from build123d import *

# Parameters (mm, degrees)
F0_R     = 1.2
F0_R_2   = 2.05
F1_DEPTH = 5.6
F2_R     = 1.6
F2_R_2   = 2.45
F3_DEPTH = 25


with BuildPart() as f1:
    # F0 (on Top) → F1 (new body)
    with BuildSketch(Plane.XY):
        with BuildLine():
            Line((31.5, 25.5), (39.5, 25.5))
            Line((39.5, 25.5), (39.5, 44.5))
            Line((39.5, 44.5), (22.808842361, 61.3844171166))
            Line((22.808842361, 61.3844171166), (0, 61.3844171166))
            Line((0, 61.3844171166), (-22.808842361, 61.3844171166))
            Line((-22.808842361, 61.3844171166), (-39.5, 44.5))
            Line((-39.5, 44.5), (-39.5, 25.5))
            Line((-39.5, 25.5), (-31.5, 25.5))
            Line((-31.5, 25.5), (-31.5, 18.901754251))
            ThreePointArc((-31.5, 18.901754251), (0, 41), (31.5, 18.901754251))
            Line((31.5, 18.901754251), (31.5, 25.5))
        make_face()
        with Locations((-35, 43)):
            Circle(F0_R, mode=Mode.SUBTRACT)
        with Locations((0, 54.8844171166)):
            Circle(F0_R_2, mode=Mode.SUBTRACT)
        with Locations((35, 43)):
            Circle(F0_R, mode=Mode.SUBTRACT)
        with BuildLine():
            Line((22.808842361, -61.3844171166), (39.5, -44.5))
            Line((39.5, -44.5), (39.5, -9.5))
            Line((39.5, -9.5), (31.5, -9.5))
            Line((31.5, -9.5), (31.5, -3.901754251))
            ThreePointArc((31.5, -3.901754251), (0, -26), (-31.5, -3.901754251))
            Line((-31.5, -3.901754251), (-31.5, -9.5))
            Line((-31.5, -9.5), (-39.5, -9.5))
            Line((-39.5, -9.5), (-39.5, -44.5))
            Line((-39.5, -44.5), (-22.808842361, -61.3844171166))
            Line((-22.808842361, -61.3844171166), (0, -61.3844171166))
            Line((0, -61.3844171166), (22.808842361, -61.3844171166))
        make_face()
        with Locations((-35, -43)):
            Circle(F0_R, mode=Mode.SUBTRACT)
        with Locations((0, -54.8844171166)):
            Circle(F0_R_2, mode=Mode.SUBTRACT)
        with Locations((35, -43)):
            Circle(F0_R, mode=Mode.SUBTRACT)
        with BuildLine():
            Line((-31.5, -9.5), (-31.5, -3.901754251))
            ThreePointArc((-31.5, -3.901754251), (-33.5, 7.5), (-31.5, 18.901754251))
            Line((-31.5, 18.901754251), (-31.5, 25.5))
            Line((-31.5, 25.5), (-39.5, 25.5))
            Line((-39.5, 25.5), (-39.5, -9.5))
            Line((-39.5, -9.5), (-31.5, -9.5))
        make_face()
        with BuildLine():
            Line((31.5, -9.5), (39.5, -9.5))
            Line((39.5, -9.5), (39.5, 25.5))
            Line((39.5, 25.5), (31.5, 25.5))
            Line((31.5, 25.5), (31.5, 18.901754251))
            ThreePointArc((31.5, 18.901754251), (32.9962119038, 13.2879184514), (33.5, 7.5))
            ThreePointArc((33.5, 7.5), (32.9962119038, 1.7120815486), (31.5, -3.901754251))
            Line((31.5, -3.901754251), (31.5, -9.5))
        make_face()
    extrude(amount=F1_DEPTH)

    # F2 (on face) → F3 (cut)
    with BuildSketch(Plane.XY.offset(5.6)):
        with Locations((-31, 38.5)):
            Circle(F2_R)
        with Locations((31, 38.5)):
            Circle(F2_R)
        with Locations((-31, -23.5)):
            Circle(F2_R)
        with Locations((31, -23.5)):
            Circle(F2_R)
        with Locations((0, 54.8844171166)):
            Circle(F2_R_2)
        with Locations((0, -54.8844171166)):
            Circle(F2_R_2)
        with BuildLine():
            ThreePointArc((10.5, 56.3844171166), (10.0606601718, 57.4450772884), (9, 57.8844171166))
            Line((9, 57.8844171166), (9, 54.8844171166))
            ThreePointArc((9, 54.8844171166), (10.0606601718, 55.3237569449), (10.5, 56.3844171166))
        make_face()
        with BuildLine():
            Line((17, 57.8844171166), (9, 57.8844171166))
            ThreePointArc((9, 57.8844171166), (10.0606601718, 57.4450772884), (10.5, 56.3844171166))
            ThreePointArc((10.5, 56.3844171166), (10.0606601718, 55.3237569449), (9, 54.8844171166))
            Line((9, 54.8844171166), (17, 54.8844171166))
            ThreePointArc((17, 54.8844171166), (15.5, 56.3844171166), (17, 57.8844171166))
        make_face()
        with BuildLine():
            Line((9, 54.8844171166), (9, 57.8844171166))
            ThreePointArc((9, 57.8844171166), (7.5, 56.3844171166), (9, 54.8844171166))
        make_face()
        with BuildLine():
            ThreePointArc((18.5, 56.3844171166), (18.0606601718, 57.4450772884), (17, 57.8844171166))
            Line((17, 57.8844171166), (17, 54.8844171166))
            ThreePointArc((17, 54.8844171166), (18.0606601718, 55.3237569449), (18.5, 56.3844171166))
        make_face()
        with BuildLine():
            Line((17, 54.8844171166), (17, 57.8844171166))
            ThreePointArc((17, 57.8844171166), (15.5, 56.3844171166), (17, 54.8844171166))
        make_face()
        with BuildLine():
            ThreePointArc((9, -57.8844171166), (10.0606601718, -57.4450772884), (10.5, -56.3844171166))
            ThreePointArc((10.5, -56.3844171166), (10.0606601718, -55.3237569449), (9, -54.8844171166))
            ThreePointArc((9, -54.8844171166), (7.5, -56.3844171166), (9, -57.8844171166))
        make_face()
        with BuildLine():
            ThreePointArc((9, -54.8844171166), (10.0606601718, -55.3237569449), (10.5, -56.3844171166))
            ThreePointArc((10.5, -56.3844171166), (10.0606601718, -57.4450772884), (9, -57.8844171166))
            Line((9, -57.8844171166), (17, -57.8844171166))
            ThreePointArc((17, -57.8844171166), (15.5, -56.3844171166), (17, -54.8844171166))
            Line((17, -54.8844171166), (9, -54.8844171166))
        make_face()
        with BuildLine():
            ThreePointArc((18.5, -56.3844171166), (18.0606601718, -55.3237569449), (17, -54.8844171166))
            ThreePointArc((17, -54.8844171166), (15.5, -56.3844171166), (17, -57.8844171166))
            ThreePointArc((17, -57.8844171166), (18.0606601718, -57.4450772884), (18.5, -56.3844171166))
        make_face()
    extrude(amount=-F3_DEPTH, mode=Mode.SUBTRACT)


solid = f1.part
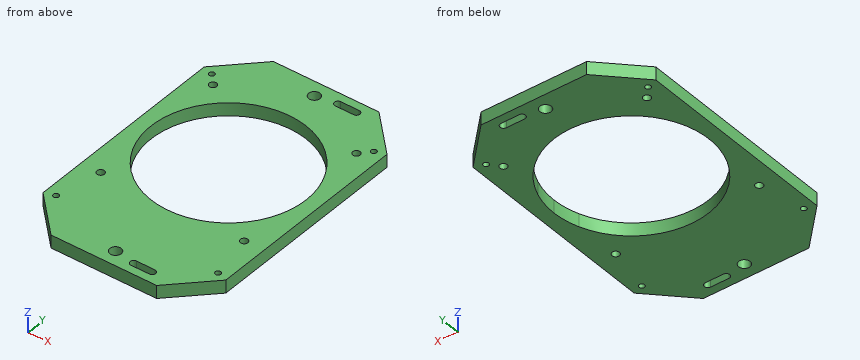
Design review of the part built by this model. Coordinates are the model's own, in mm. Coordinates: 2 decimals unless noted, no trailing zeros. Write each loop counter-clockwise with the first axis right and the second up, starting at its lowest first coordinate (ties: lowest second). Pieces come first, ordered by that corner, then holes. Notation, with made-up numbers: (-29.75, -31.75) - (-13.75, -31.75) arc R20 cw to (-13.75, -22.75) - close; hole circle Ø11 at (-1, 77). An arc over 180 degrees is marked (long way). One line per item, written item: value.
1) Add section A-A (x = 0). State the section outline as (y, z) points, plus the area to 3 significant figures.
Answer sheet:
outline: (-61.38, 0) - (-57.33, 0) - (-57.33, 5.6) - (-61.38, 5.6) - close; (-52.43, 0) - (-26, 0) - (-26, 5.6) - (-52.43, 5.6) - close; (41, 0) - (52.43, 0) - (52.43, 5.6) - (41, 5.6) - close; (57.33, 0) - (61.38, 0) - (61.38, 5.6) - (57.33, 5.6) - close
area: 257 mm2
2) Add section B-B (z = 1.85). Give the number of separate pieces and of enclosed holes in the cut face, plus the area to 3 significant figures.
Answer sheet:
separate pieces: 1
enclosed holes: 13
area: 5,460 mm2
3) Add section D-D (x = 26). State the section outline as (y, z) points, plus the area to 3 significant figures.
Answer sheet:
outline: (-58.16, 0) - (-13.62, 0) - (-13.62, 5.6) - (-58.16, 5.6) - close; (28.62, 0) - (58.16, 0) - (58.16, 5.6) - (28.62, 5.6) - close
area: 415 mm2
4) Add section C-C (y = 43). State the section outline as (x, z) points, plus the area to 3 significant figures.
Answer sheet:
outline: (-39.5, 0) - (-36.2, 0) - (-36.2, 5.6) - (-39.5, 5.6) - close; (-33.8, 0) - (33.8, 0) - (33.8, 5.6) - (-33.8, 5.6) - close; (36.2, 0) - (39.5, 0) - (39.5, 5.6) - (36.2, 5.6) - close
area: 416 mm2
5) Insertion check: pin 1 (3 mm diameter, centred on x = 27, z = 1, fed in from +Y); pin 2 (1.9 mm diameter, centred on x = -35, y = 43, fed in from -Z). Each pin has a flat end and moves straight along its axis. Give the tip position at first contact, or say it passes through.
Answer sheet:
pin 1: stops at y = 58.66
pin 2: passes through
6) To check wall thickness, follow probe 1 along Y at (x, z) = (0, 2.2); probe 2 along Y at (x, z) = (17, 4.8); probe 3 along X at (y, z) = (56, 0.45). State the ranges of each line that lie inside material, in increasing order.
Answer sheet:
probe 1: y = -61.38 to -57.33, -52.43 to -26, 41 to 52.43, 57.33 to 61.38
probe 2: y = -61.38 to -57.88, -54.88 to -21.37, 36.37 to 54.88, 57.88 to 61.38
probe 3: x = -28.13 to -2.18, 2.18 to 7.55, 18.45 to 28.13
